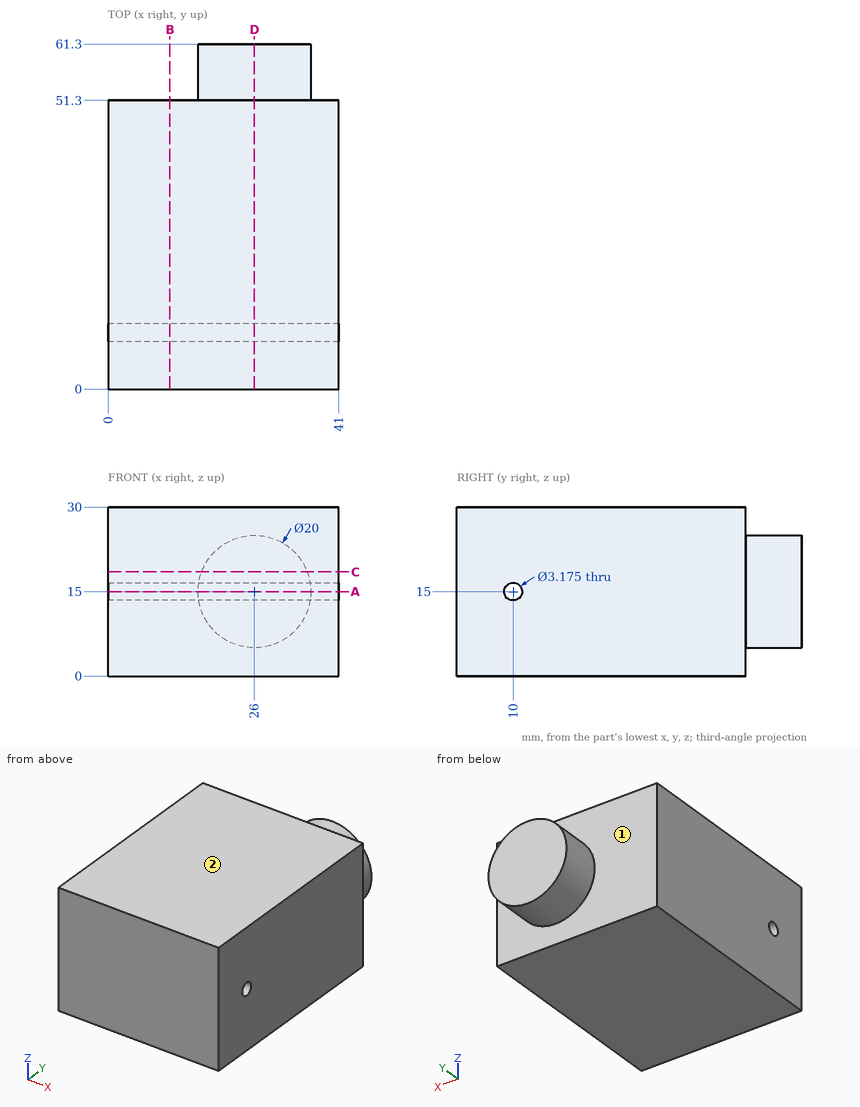
Check sheet for the drawn part. Datum: minimum x, y, z corner. Units: mm. A direction names the side the tool comes from. Give positions to 0.01 mm unless a question says otherwise; leave off trailing zeros. Order: outer loops, then holes, each group sorted by start corner. A loop starts at its lowest first (then second) coordinate and runs counter-clockwise, first axis right, second up.
1. Scan lines: line 1 (Y direction, x = 23, z = 15); line 2 (Y direction, x = 11, z = 15); line 3 (Y direction, x = 10, z = 9). Record each from-to range of solid material in increasing order.
Completed:
line 1: y = 0 to 8.41, 11.59 to 61.3
line 2: y = 0 to 8.41, 11.59 to 51.3
line 3: y = 0 to 51.3
2. Sectioned sample at A-A (z = 15). Record the boundary of the cut face in (x, y), then the cut area to 3 significant figures.
Completed:
outline: (0, 0) - (41, 0) - (41, 8.41) - (0, 8.41) - close; (0, 11.59) - (41, 11.59) - (41, 51.3) - (36, 51.3) - (36, 61.3) - (16, 61.3) - (16, 51.3) - (0, 51.3) - close
area: 2,170 mm2
3. Depth check by flat-ended pin: pin 1 (12 mm diameter, centred on x = 36, y = 45, fed in from -Z); pin 2 (3 mm diameter, centred on x = 17, z = 25.5, fed in from +Y). Enter the tip coordinate at first touch or a pass-through.
Completed:
pin 1: stops at z = 0
pin 2: stops at y = 51.3
4. Sectioned sample at D-D (x = 26). Record the boundary of the cut face in (y, z) (1 decimal).
Completed:
outline: (0, 0) - (51.3, 0) - (51.3, 5) - (61.3, 5) - (61.3, 25) - (51.3, 25) - (51.3, 30) - (0, 30) - close; hole circle Ø3.2 at (10, 15)
5. Access from +Z, -Z, +X, -X, +Y, -Y to the whole of each face (thin tool, end or side, straight path). Record for the marked faces 1 and 2.
Completed:
face 1: +Y
face 2: +Z, +X, -X, +Y, -Y
6. Sectioned sample at C-C (z = 18.5). Record the boundary of the cut face in (x, y), then the cut area to 3 significant figures.
Completed:
outline: (0, 0) - (41, 0) - (41, 51.3) - (35.37, 51.3) - (35.37, 61.3) - (16.63, 61.3) - (16.63, 51.3) - (0, 51.3) - close
area: 2,290 mm2
7. Sectioned sample at B-B (x = 11). Record the boundary of the cut face in (y, z) (1 decimal), then the cut area to 3 significant figures.
Completed:
outline: (0, 0) - (51.3, 0) - (51.3, 30) - (0, 30) - close; hole circle Ø3.2 at (10, 15)
area: 1,530 mm2
